For this review, take the finished solid that the model builds, in its own axes (mm). A direction names the side the tool comes from. Round coordinates to 2 decimals unless told otherwise and drop trailing zeros. Loops run counter-clockwise (first coordinate to the right, second up) from the corner with the lowest first, then second, coordinate; pieces in that order, holes last.
1) Take a section at C-C (z = 0). State the section outline as (x, y) points.
2) Take a section at D-D (y = -22.5). State the section outline as (x, z) points, then the cut area to 3 significant figures.
3) Take a section at B-B (x = 100). State the section outline as (y, z) points.
4) Tool access review of faces 1 (the flat face through (188, 5, -1)), 2 (the flat face through (188, -5, -1)), 3 (the flat face through (-80.53, -58.04, 0.52)): name each direction out of +Z, -Z, +X, -X, +Y, -Y from which nothing blocks a thin tool from reaching the whole face with its end or side.
5) Insertion check: pin 1 (10 mm diameter, centred on y = -9, z = 1, fed in from -X); pin 2 (6 mm diameter, centred on y = -19.5, z = 20, fed in from +X); pin 3 (5.5 mm diameter, centred on y = 8, z = 7, fed in from +X); pin 4 (3 mm diameter, centred on x = 99.5, y = 10.5, fed in from -Z). Each pin has a flat end and moves straight along its axis. Give the tip position at first contact, or say it passes through.
6) Take a section at A-A (y = 0). State the section outline as (x, z) points.
7) Mouldability with a two-part tool opening along X and no side actions: class faces 4 (the flat face through (-138, -80, 5)), 5 (the flat face through (-151.377, -87.236, -21.022)), 6 (the cylindrical face through (12.19, -48.49, 0.52)) as pulls with the +X half, pulls with the -X half, needs draft (parallel to the pull), parting line crosses it, or undercut.
8) Wall thickness on L1, parallel to Z at x = 100, y = -2; L2, parallel to Y at x = 0, z = 0; L3, parallel to X at y = -33.5, z = -25: over which ranges is each line inside the solid? List them lowest first.
```python
from build123d import *

# Parameters (mm, degrees)
IZIM1_R                     = 50
IZIM1_R_2                   = 37.5
IZIM1_W                     = 25
IZIM1_H                     = 10
Y_KSEKLIK_EKSTR_ZYON1_DEPTH = 37.5
Y_KSEKLIK_EKSTR_ZYON2_DEPTH = 10
IZIM3_R                     = 12.5
KES_EKSTR_ZYON1_DEPTH       = 10
IZIM4_R                     = 12.5
KES_EKSTR_ZYON2_DEPTH       = 107.017280086
KES_EKSTR_ZYON3_DEPTH       = 200.403403757


with BuildPart() as part:
    # Çizim1 → Yükseklik-Ekstrüzyon1 (new body, symmetric)
    with BuildSketch(Plane.XY):
        with BuildLine():
            Line((-156.306807514, -78.69677201), (-146.306807514, -96.017280086))
            Line((-146.306807514, -96.017280086), (-37.426406871, -33.155151466))
            ThreePointArc((-37.426406871, -33.155151466), (-43.301270189, -25), (-47.426406871, -15.83464339))
            Line((-47.426406871, -15.83464339), (-156.306807514, -78.69677201))
        make_face()
        Circle(IZIM1_R)
        Circle(IZIM1_R_2, mode=Mode.SUBTRACT)
        with BuildLine():
            ThreePointArc((50, 0), (49.74680765, -5.0254481), (48.989794856, -10))
            Line((48.989794856, -10), (150, -10))
            Line((150, -10), (150, -5))
            Line((150, -5), (150, 5))
            Line((150, 5), (150, 10))
            Line((150, 10), (48.989794856, 10))
            ThreePointArc((48.989794856, 10), (49.74680765, 5.0254481), (50, 0))
        make_face()
        with Locations((162.5, 0)):
            Rectangle(IZIM1_W, IZIM1_H)
    extrude(amount=Y_KSEKLIK_EKSTR_ZYON1_DEPTH, both=True)

    # Çizim2 → Yükseklik-Ekstrüzyon2 (add)
    with BuildSketch(Plane(origin=(0, 5, 0), x_dir=(1, 0, 0), z_dir=(0, 1, 0))):
        with BuildLine():
            Line((175, 37.5), (175, -37.5))
            ThreePointArc((175, -37.5), (212.5, 0), (175, 37.5))
        make_face()
    extrude(amount=-Y_KSEKLIK_EKSTR_ZYON2_DEPTH)

    # Çizim3 → Kes-Ekstrüzyon1 (cut)
    with BuildSketch(Plane(origin=(0, 5, 0), x_dir=(1, 0, 0), z_dir=(0, 1, 0))):
        with Locations((175, 0)):
            Circle(IZIM3_R)
    extrude(amount=-KES_EKSTR_ZYON1_DEPTH, mode=Mode.SUBTRACT)

    # Çizim4 → Kes-Ekstrüzyon2 (cut, through all)
    with BuildSketch(Plane(origin=(0, 10, 0), x_dir=(1, 0, 0), z_dir=(0, 1, 0))):
        with Locations((100, 0)):
            Circle(IZIM4_R)
    extrude(amount=-KES_EKSTR_ZYON2_DEPTH, mode=Mode.SUBTRACT)

    # Çizim5 → Kes-Ekstrüzyon3 (cut, through all)
    with BuildSketch(Plane(origin=(-5, 8.660254038, 0), x_dir=(0.866025404, 0.5, 0), z_dir=(-0.5, 0.866025404, 0))):
        with BuildLine():
            Line((-174.714052097, 5), (-174.714052097, -5))
            Line((-174.714052097, -5), (-144.078968828, -5))
            ThreePointArc((-144.078968828, -5), (-104.714052097, 0), (-144.078968828, 5))
            Line((-144.078968828, 5), (-174.714052097, 5))
        make_face()
    extrude(amount=-KES_EKSTR_ZYON3_DEPTH, mode=Mode.SUBTRACT)


solid = part.part
```
Response:
1. outline: (-95.69, -43.7) - (-85.69, -61.02) - (-37.43, -33.16) arc R50 ccw to (48.99, -10) - (87.5, -10) - (87.5, 10) - (48.99, 10) arc R50 ccw (long way) to (-47.43, -15.83) - close; (112.5, -10) - (150, -10) - (150, -5) - (162.5, -5) - (162.5, 5) - (150, 5) - (150, 10) - (112.5, 10) - close; (187.5, -5) - (212.5, -5) - (212.5, 5) - (187.5, 5) - close; hole circle Ø75 at (0, 0)
2. outline: (-58.97, -37.5) - (-30, -37.5) - (-30, 37.5) - (-58.97, 37.5) - close; (30, -37.5) - (44.65, -37.5) - (44.65, 37.5) - (30, 37.5) - close
2. area: 3,270 mm2
3. outline: (-10, -37.5) - (10, -37.5) - (10, -12.5) - (-10, -12.5) - close; (-10, 12.5) - (10, 12.5) - (10, 37.5) - (-10, 37.5) - close
4. face 1: +Z, -Z, +X, +Y
4. face 2: +Z, -Z, +X, -Y
4. face 3: +Z, -Z, -Y
5. pin 1: stops at x = -49.84
5. pin 2: stops at x = 47.2
5. pin 3: stops at x = 150
5. pin 4: stops at z = -37.5
6. outline: (-50, -37.5) - (-37.5, -37.5) - (-37.5, 37.5) - (-50, 37.5) - close; (37.5, -37.5) - (175, -37.5) arc R37.5 ccw to (175, 37.5) - (37.5, 37.5) - close; hole circle Ø25 at (100, 0); hole circle Ø25 at (175, 0)
7. face 4: needs draft
7. face 5: pulls with the -X half
7. face 6: undercut
8. L1: z = -37.5 to -12.5, 12.5 to 37.5
8. L2: y = -50 to -37.5, 37.5 to 50
8. L3: x = -78.02 to -38.02, -37.12 to -16.85, 16.85 to 37.12
